from build123d import *

# Parameters (mm, degrees)
F1_DEPTH = 3.175
F2_R     = 20.6375
F2_R_2   = 1.7272
F3_DEPTH = 3.175


with BuildPart() as f1:
    # F0 (on Top) → F1 (new body)
    with BuildSketch(Plane.XY):
        Polygon((304.8, -344.886255), (304.8, 0), (284.382272, 76.2), (228.6, 131.982272), (152.4, 152.4), (76.2, 131.982272), (20.417728, 76.2), (0, 0), (0, -344.886255), (20.417728, -421.086255), (76.2, -476.868526), (152.4, -497.286255), (228.6, -476.868526), (284.382272, -421.086255), align=None)
    extrude(amount=F1_DEPTH)

    # F2 (on face) → F3 (cut, through all)
    with BuildSketch(Plane.XY.offset(3.175)):
        with Locations((227.258907, 30.807116)):
            Circle(F2_R)
        with Locations((88.192595, -33.361206)):
            Circle(F2_R_2)
        with Locations((214.795642, -33.977575)):
            Circle(F2_R_2)
        with Locations((197.890157, 1.438366)):
            Circle(F2_R_2)
        with Locations((256.627657, 1.438366)):
            Circle(F2_R_2)
        with Locations((256.627657, 60.175866)):
            Circle(F2_R_2)
        with Locations((197.890157, 60.175866)):
            Circle(F2_R_2)
        with Locations((213.92522, -212.763443)):
            Circle(F2_R_2)
        with Locations((87.322173, -212.147074)):
            Circle(F2_R_2)
        with Locations((152.542099, -468.099017)):
            Circle(F2_R_2)
        with Locations((255.188616, -366.447129)):
            Circle(F2_R_2)
        with Locations((153.536729, -263.800611)):
            Circle(F2_R_2)
        with Locations((50.890211, -365.452499)):
            Circle(F2_R_2)
        with Locations((152.248171, 121.214165)):
            Circle(F2_R_2)
        with Locations((151.93902, 57.714165)):
            Circle(F2_R_2)
        with Locations((68.055466, 82.76303)):
            Circle(F2_R_2)
        with Locations((233.581526, 82.76303)):
            Circle(F2_R_2)
        with Locations((68.055466, -427.649284)):
            Circle(F2_R_2)
        with Locations((233.581526, -427.649284)):
            Circle(F2_R_2)
    extrude(amount=-F3_DEPTH, mode=Mode.SUBTRACT)


solid = f1.part
Geometry: final body of the model. Coordinates: model frame, mm. Give positions to 0.01 mm unless a question says otherwise; leave off trailing zeros. Order: outer loops, then holes, each group sorted by start corner. A loop starts at its lowest first (then second) coordinate and runs counter-clockwise, first axis right, second up. Notation, with made-up numbers: (11, -18) -> (25, -18) arc R19 ccw to (25, -8) -> close; hole circle Ø6 at (70.5, -32.5). An arc over 180 degrees is marked (long way). Write each question's results on one line, items separated by ' | '.
1) Cut plane B-B (y = -455.5). Output: boundary loops of the cut face in (x, z) (3 decimals), and give its area (3 significant figures).
Geometry says:
outline: (54.831, 0) -> (249.969, 0) -> (249.969, 3.175) -> (54.831, 3.175) -> close | area: 620 mm²
2) Cut plane C-C (x = 180). Output: boundary loops of the cut face in (y, z) (3 decimals).
Geometry says:
outline: (-489.891, 0) -> (145.005, 0) -> (145.005, 3.175) -> (-489.891, 3.175) -> close
3) Draft query along X for faces 1 (the face through (189.97, -487.22, 1.57)), 2 (the face through (150, -168, 3.175)), 3 (the face through (113.767, -486.934, 1.565)), 4 (the face through (246.32, 22.9, 1.61)). Return one class per face: released by +X, released by -X, zero draft, split by the parting line, or undercut.
Geometry says:
face 1: released by +X | face 2: zero draft | face 3: released by -X | face 4: undercut
4) Cut plane A-A (z = 2.6). Give the number of separate pieces and of enclosed holes in the cut face, and give its area (3 significant figures).
Geometry says:
separate pieces: 1 | enclosed holes: 19 | area: 173,000 mm²
5) Line query: line 1 along Y through (x, z) = (240.5, 0.45); line 2 along X through (y, z) = (25, 2.05); line 3 along X through (y, z) = (43, 0.25). Output: solid intervals per line, ascending.
Geometry says:
line 1: y = -464.97 to 14.98, 46.64 to 120.08 | line 2: x = 6.7 to 207.46, 247.06 to 298.1 | line 3: x = 11.52 to 210.61, 243.91 to 293.28
